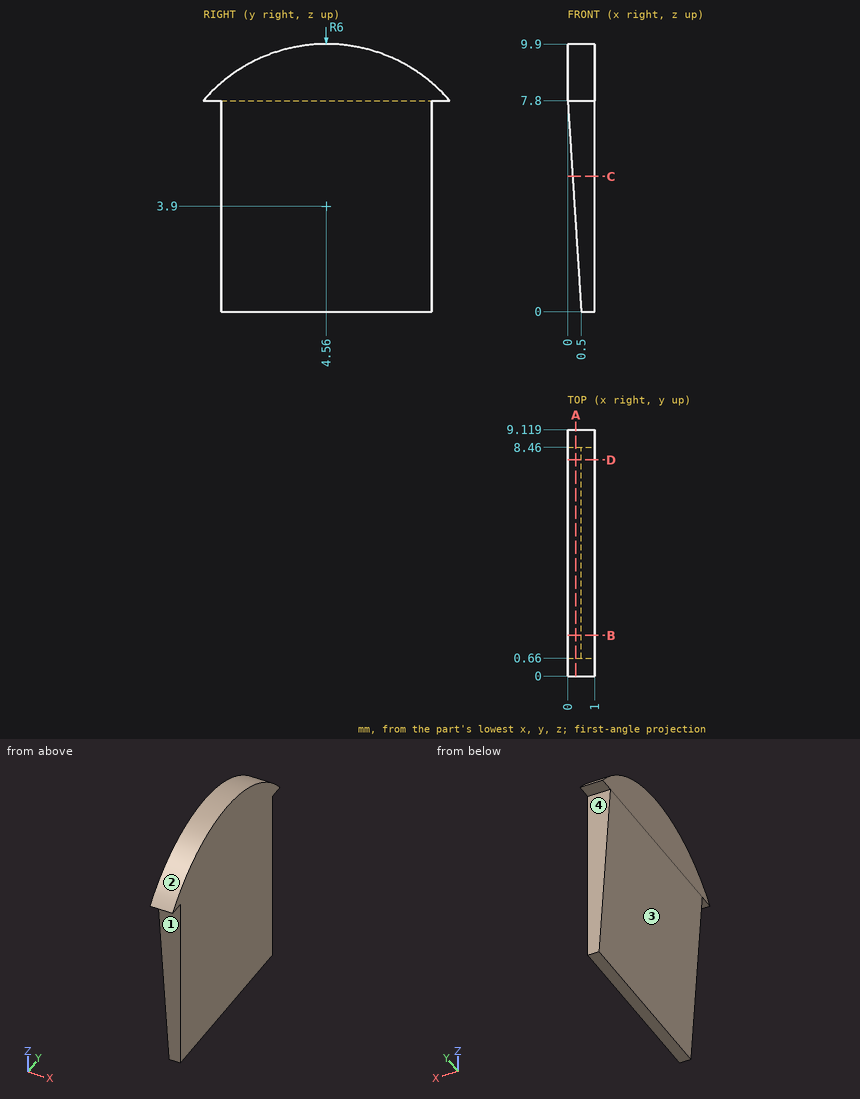
Print and shaded views of the part. All mm, measured from the part's lowest x, y and z. Give positions to 0.01 mm unless a question says otherwise; leave off trailing zeros. Loops run counter-clockwise (first coordinate to the right, second up) from the corner with the lowest first, then second, coordinate; pieces in that order, holes last. Notation, with made-up numbers: (5, -14) -> (12, -14) arc R14 cw to (12, -1) -> close; hole circle Ø7 at (31.5, 34.25). An arc over 180 degrees is marked (long way). Answer in a Markdown table with one row per item.
Item 1: Flat gauge pins, fed straight in: P1, Ø1.5, axis at y = 3.5, z = 4.5, coming from the -X side; P2, Ø0.5, axis at x = 0.5, z = 3.5, coming from the +Y side. Where does each tip first touch, or does it go through?
Findings below:
| item | result |
|---|---|
| P1 | stops at x = 0.16 |
| P2 | stops at y = 8.46 |
Item 2: Slice it at B-B on y = 1.5. Write the cut outline in (x, z).
Findings below:
| item | result |
|---|---|
| outline | (0, 7.8) -> (0.5, 0) -> (1, 0) -> (1, 9.06) -> (0, 9.06) -> close |
Item 3: Slice it at A-A on x = 0.3. Write the cut outline in (y, z), plus the area to 3 significant figures.
Findings below:
| item | result |
|---|---|
| outline | (0, 7.8) -> (0.66, 7.8) -> (0.66, 3.12) -> (8.46, 3.12) -> (8.46, 7.8) -> (9.12, 7.8) arc R6 ccw to start |
| area | 49.8 mm² |
Item 4: Slice it at D-D on y = 8. Write the cut outline in (x, z) (1 decimal).
Findings below:
| item | result |
|---|---|
| outline | (0, 7.8) -> (0.5, 0) -> (1, 0) -> (1, 8.8) -> (0, 8.8) -> close |
Item 5: Slice it at C-C on z = 5. Write the cut outline in (x, y).
Findings below:
| item | result |
|---|---|
| outline | (0.18, 0.66) -> (1, 0.66) -> (1, 8.46) -> (0.18, 8.46) -> close |
Item 6: Mould opens along Y. For the marked faces 1, 2, 3 and 4 say: pulls with the +Y half, pulls with the -Y half, needs draft (parallel to the pull), parting line crosses it, or undercut.
Findings below:
| item | result |
|---|---|
| face 1 | pulls with the -Y half |
| face 2 | parting line crosses it |
| face 3 | needs draft |
| face 4 | pulls with the +Y half |
Item 7: Probe line 1 along Y through (x, z) = (0.15, 6.25); line 2 along X through (y, z) = (2, 2.75); line 3 along X through (y, z) = (5, 5.5). List the from-to ranges inside material, lowest first. Write a range as [from, to].
Findings below:
| item | result |
|---|---|
| line 1 | y = [0.66, 8.46] |
| line 2 | x = [0.32, 1] |
| line 3 | x = [0.15, 1] |
